Read the model definition and answer for the solid it produces. Units are mm, in the model's axes. Face numbers are marked on the shaded views. A direction names the side the tool comes from. Give positions to 0.01 mm unless a question says otherwise; leave off trailing zeros. Order: outer loops, then holes, each group sorted by start corner. A loop starts at its lowest first (then second) coordinate and runs counter-clockwise, first axis right, second up. Notation, with made-up numbers: (71.5, -5) - (126.5, -5) arc R16 ccw to (126.5, 25) - close; hole circle Ø3 at (81, 19). An arc over 180 degrees is marked (long way). Return JSON: item names as keys, results as strings.
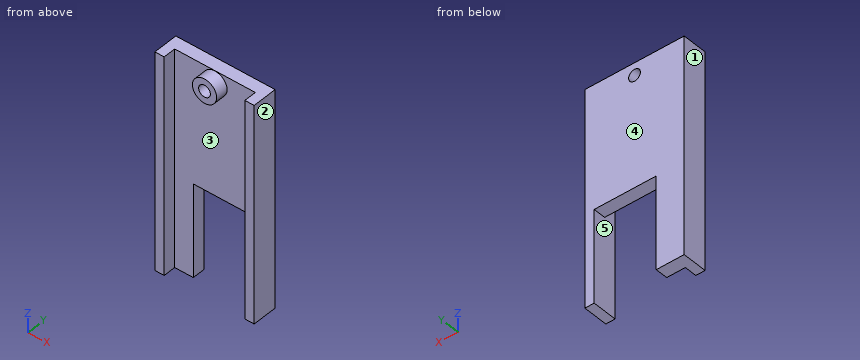
Autodesk Inventor part; units mm, degrees
ref_plane "YZ Plane" through (0, 0, 0) normal (1, 0, 0) x (0, 1, 0)
ref_plane "XZ Plane" through (0, 0, 0) normal (0, 1, 0) x (-1, 0, 0)
ref_plane "XY Plane" through (0, 0, 0) normal (0, 0, 1) x (1, 0, 0)
sketch "Skizze1" plane through (0, 0, 0) normal (0, 1, 0) x (-1, 0, 0)
  line L0 (0, 0) -> (0, -35)
  line L1 (0, -35) -> (-4.5, -35)
  line L2 (-4.5, -35) -> (-4.5, -20)
  line L3 (-4.5, -20) -> (-14.5, -20)
  line L4 (-14.5, -20) -> (-14.5, -35)
  line L5 (-14.5, -35) -> (-16, -35)
  line L6 (-16, -35) -> (-16, 0)
  line L7 (-16, 0) -> (0, 0)
  circle A0 centre (-8, -2) radius 0.95
  point P0 (-8, 0)
  dimension "d0" = 16
  dimension "d1" = 1.9
  dimension "d2" = 2
  dimension "d4" = 33
  dimension "d5" = 15
  dimension "d6" = 10
  dimension "d7" = 4.5
extrude "Extrusion1" add sketch "Skizze1" against normal blind 2
sketch "Skizze2" plane through (0, -2, 0) normal (0, -1, 0) x (1, 0, 0)
  line L0 (16, -35) -> (16, 0)
  line L1 (16, 0) -> (0, 0)
  line L2 (0, 0) -> (0, -35)
  line L3 (0, -35) -> (4.5, -35)
  line L4 (4.5, -35) -> (4.5, -20)
  line L5 (4.5, -20) -> (14.5, -20)
  line L6 (14.5, -20) -> (14.5, -35)
  line L7 (14.5, -35) -> (16, -35)
  circle A0 centre (8, -2) radius 0.95
  circle A1 centre (8, -2) radius 1.95
  line L8 (0, 0) -> (16, 0)
  line L9 (1.5, 0) -> (1.5, -35)
  line L10 (0, -35) -> (4.5, -35)
  line L11 (14.5, -35) -> (16, -35)
  line L12 (14.5, -20) -> (14.5, 0)
  point P0 (14.5, 0)
  dimension "d10" = 1
  dimension "d11" = 1.5
extrude "Extrusion2" add sketch "Skizze2" along normal blind 2 contours L7 L6 L12 L1 L0 | L9 L3 L2 L1 | A1
properties part number "power_halterung"
Q1. A cutting plane is placed at D-D (y = -1.5). Write down the section's boundary in (x, z).
Values:
{"outline": "(0, -35) - (4.5, -35) - (4.5, -20) - (14.5, -20) - (14.5, -35) - (16, -35) - (16, 0) - (0, 0) - close; hole circle Ø1.9 at (8, -2)"}
Q2. A cutting plane is placed at A-A (y = -3.5). Write down the section's boundary in (x, z).
Values:
{"outline": "(0, -35) - (1.5, -35) - (1.5, 0) - (0, 0) - close; circle Ø3.9 at (8, -2); (14.5, -35) - (16, -35) - (16, 0) - (14.5, 0) - close; hole circle Ø1.9 at (8, -2)"}
Q3. Given pin 1 (2 mm diameter, centred on x = 10.5, y = -1.5, fed in from -Z); pin 2 (8 mm diameter, centred on x = 7, z = -30, fed in from -Y), each flat-ended and moving along its own axis, determine where each tip first touches the part or whether it passes through.
Values:
{"pin 1": "stops at z = -20", "pin 2": "stops at y = -2"}
Q4. A cutting plane is placed at C-C (x = 8). Write down the section's boundary in (y, z), and give its area (3 significant figures).
Values:
{"outline": "(-4, -3.95) - (-2, -3.95) - (-2, -20) - (0, -20) - (0, -2.95) - (-4, -2.95) - close; (-4, -1.05) - (0, -1.05) - (0, 0) - (-2, 0) - (-2, -0.05) - (-4, -0.05) - close", "area": "40.2 mm²"}
Q5. A cutting plane is placed at B-B (z = -2). Write down the section's boundary in (x, y).
Values:
{"outline": "(0, -4) - (1.5, -4) - (1.5, -2) - (6.05, -2) - (6.05, -4) - (7.05, -4) - (7.05, 0) - (0, 0) - close; (8.95, -4) - (9.95, -4) - (9.95, -2) - (14.5, -2) - (14.5, -4) - (16, -4) - (16, 0) - (8.95, 0) - close"}
Q6. For the marked faces 4 and 5, determine the directions among +Z, -Z, +X, -X, +Y, -Y from which every point of the face is accessible in a straight line to the end or side of a thin tool.
Values:
{"face 4": "+Z, -Z, +X, -X, +Y", "face 5": "-Z, -Y"}
Q7. Consider L1, parallel to X at y = -2.35, z = -11; L2, parallel to X at y = -1.9, z = -2; L3, parallel to Z at x = 8, y = -1.95. Determine where each line is inside the solid, lowest interval first.
Values:
{"L1": "x = 0 to 1.5, 14.5 to 16", "L2": "x = 0 to 7.05, 8.95 to 16", "L3": "z = -20 to -2.95, -1.05 to 0"}
Q8. Determine the mould class of the marked faces 1, 2 and 3 for opening direction X: released by +X, released by -X, zero draft, split by the parting line, or undercut.
Values:
{"face 1": "released by -X", "face 2": "released by +X", "face 3": "undercut"}
